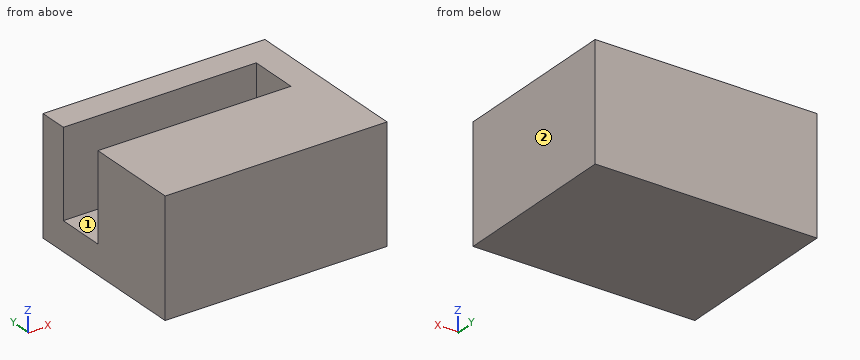
Autodesk Inventor part; units mm, degrees
ref_plane "YZ Plane" through (0, 0, 0) normal (1, 0, 0) x (0, 1, 0)
ref_plane "XZ Plane" through (0, 0, 0) normal (0, 1, 0) x (-1, 0, 0)
ref_plane "XY Plane" through (0, 0, 0) normal (0, 0, 1) x (1, 0, 0)
sketch "base" plane through (0, 0, 0) normal (0, 1, 0) x (-1, 0, 0)
  line L0 (-11.5, 6) -> (11.5, 6)
  line L1 (11.5, 6) -> (11.5, -6)
  line L2 (11.5, -6) -> (-11.5, -6)
  line L3 (-11.5, -6) -> (-11.5, 6)
  line L4 (-11.5, 6) -> (11.5, -6) construction
  line L5 (11.5, 6) -> (-11.5, -6) construction
  point P0 (0, 0)
  dimension "d0" = 23
  dimension "d1" = 12
extrude "Extrusion1" add sketch "base" along normal blind 18
sketch "Sketch3" plane through (-11.5, 0, 6) normal (0, 0, 1) x (1, 0, 0)
  line L0 (20, 9.9) -> (0, 9.9)
  line L1 (0, 9.9) -> (0, 15)
  line L2 (0, 15) -> (20, 15)
  line L3 (20, 15) -> (20, 9.9)
  line L4 (0, 0) -> (0, 18)
  line L5 (0, 18) -> (23, 18)
  line L6 (23, 0) -> (23, 18)
  point P0 (11.5, 0)
  dimension "d9" = 5.1
  dimension "d10" = 3
  dimension "d11" = 3
extrude "Extrusion3" cut sketch "Sketch3" against normal blind 9
equation "\"d11\" = d10"
properties part number "peg_TR"
Can you work these out from the model? Positions are in its coordinate system, mm. Face numbers are marked on the shaded views. A direction names the side the tool comes from. Coordinates: 2 decimals unless noted, no trailing zeros. Loops run counter-clockwise (first coordinate to the right, second up) from the corner with the lowest first, then second, coordinate; pieces in that order, holes last. Notation, with made-up numbers: M 69,-34 L 99,-34 A17 cw 99,-18 Z; hole C 67.5,-28 d7. An arc over 180 degrees is marked long. Return JSON: item names as keys, results as strings. Group by question number.
Item 1: Imagine slicing it at C-C (y = 13.5). Please give me the cut outline in (x, z).
Item 2: If I drill on L1, parallel to Y at x = -2.75, z = 4.5; L2, parallel to Z at x = -8, y = 14.25; L3, parallel to X at y = 10.25, z = 5.75, over which ranges is the centre line in solid material (lowest first)? Write a range as from..to.
Item 3: Imagine slicing it at B-B (z = -1.5). Please give me the cut outline in (x, y), and give its area (3 significant figures).
Item 4: I'm going to push flat-ended pins straight in: pin 1 Ø5.5 at (x, y) = (-3, 12) entering from +Z; pin 2 Ø4 at (y, z) = (12.5, 3.5) entering from -X. Where does each tip first touch, or does it pass through?
Item 5: On a 3-axis mill with a long thin cutter (end or side, diameter ignored), from which of +Z, -Z, +X, -X, +Y, -Y can I reach the whole of each face in a straight line? I mean the marked faces 1 and 2. Say none if no direction works.
Item 6: Imagine slicing it at A-A (x = -0.75). Please give me the cut outline in (y, z).
Verdict:
{
 "1": {"outline": "M -11.5,-6 L 11.5,-6 L 11.5,6 L 8.5,6 L 8.5,-3 L -11.5,-3 Z"},
 "2": {"L1": "y = 0..9.9, 15..18", "L2": "z = -6..-3", "L3": "x = 8.5..11.5"},
 "3": {"outline": "M -11.5,0 L 11.5,0 L 11.5,18 L -11.5,18 L -11.5,15 L 8.5,15 L 8.5,9.9 L -11.5,9.9 Z", "area": "312 mm^2"},
 "4": {"pin 1": "stops at z = 6", "pin 2": "stops at x = 8.5"},
 "5": {"face 1": "+Z, -X", "face 2": "+Z, -Z, +X, +Y, -Y"},
 "6": {"outline": "M 0,-6 L 18,-6 L 18,6 L 15,6 L 15,-3 L 9.9,-3 L 9.9,6 L 0,6 Z"}
}
